from build123d import *

# Parameters (mm, degrees)
F0_W      = 50.8
F0_H      = 57.15
F1_DEPTH  = 3.175
F2_W      = 50.8
F2_H      = 3.175
F3_DEPTH  = 88.9
F4_W      = 50.8
F4_H      = 3.175
F5_DEPTH  = 88.9
F6_W      = 50.8
F6_H      = 88.9
F7_DEPTH  = 3.175
F8_W      = 57.15
F8_H      = 92.075
F9_DEPTH  = 3.175
F11_W     = 44.45
F11_H     = 3.175
F12_DEPTH = 88.9
F10_W     = 3.175
F10_H     = 50.8
F13_DEPTH = 88.9


with BuildPart() as f1:
    # F0 (on Top) → F1 (new body)
    with BuildSketch(Plane.XY):
        Rectangle(F0_W, F0_H)
    extrude(amount=F1_DEPTH)

    # F2 (on face) → F3 (join)
    with BuildSketch(Plane.XY.offset(3.175)):
        with Locations((0, 26.9875)):
            Rectangle(F2_W, F2_H)
    extrude(amount=F3_DEPTH)

    # F4 (on face) → F5 (join)
    with BuildSketch(Plane.XY.offset(3.175)):
        with Locations((0, -26.9875)):
            Rectangle(F4_W, F4_H)
    extrude(amount=F5_DEPTH)

    # F6 (on face) → F7 (join)
    with BuildSketch(Plane(origin=(-25.4, 0, 0), x_dir=(0, -1, 0), z_dir=(-1, 0, 0))):
        with Locations((0, 47.625)):
            Rectangle(F6_W, F6_H)
    extrude(amount=-F7_DEPTH)

    # F8 (on face) → F9 (join)
    with BuildSketch(Plane.YZ.offset(25.4)):
        with Locations((0, 46.0375)):
            Rectangle(F8_W, F8_H)
    extrude(amount=-F9_DEPTH)

    # F11 (on face) → F12 (join)
    with BuildSketch(Plane.XY.offset(3.175)):
        Rectangle(F11_W, F11_H)
    extrude(amount=F12_DEPTH)

    # F10 (on face) → F13 (join)
    with BuildSketch(Plane.XY.offset(3.175)):
        Rectangle(F10_W, F10_H)
    extrude(amount=F13_DEPTH)


solid = f1.part
Can you work these out from the model? Positions are in its coordinate system, mm. A direction names the side the tool comes from. Give positions to 0.01 mm unless a question says otherwise; leave off trailing zeros. Loops run counter-clockwise (first coordinate to the right, second up) from the corner with the lowest first, then second, coordinate; pieces in that order, holes last. Notation, with made-up numbers: (60.25, -9.75) -> (65.25, -9.75) arc R14 ccw to (65.25, 9.25) -> close; hole circle Ø5 at (46, -10). An arc over 180 degrees is marked (long way). Return JSON: item names as keys, results as strings.
Q1. On a 3-axis mill with a long thin cutter (end or side, diameter ignored), from which of +Z, -Z, +X, -X, +Y, -Y can I reach the whole of each face in a straight line? I mean faces 1 (the face through (-1.588, 13, 47)), 2 (the face through (0, -28.575, 45)). Say none if no direction works.
Checks:
{"face 1": "+Z", "face 2": "+Z, -Z, +X, -X, -Y"}
Q2. I want a section at A-A, the plane z = 83. List the corners of the cut face in (x, y) for me (1 decimal).
Checks:
{"outline": "(-25.4, -28.6) -> (25.4, -28.6) -> (25.4, 28.6) -> (-25.4, 28.6) -> close; hole (-22.2, -25.4) -> (-1.6, -25.4) -> (-1.6, -1.6) -> (-22.2, -1.6) -> close; hole (-22.2, 1.6) -> (-1.6, 1.6) -> (-1.6, 25.4) -> (-22.2, 25.4) -> close; hole (1.6, -25.4) -> (22.2, -25.4) -> (22.2, -1.6) -> (1.6, -1.6) -> close; hole (1.6, 1.6) -> (22.2, 1.6) -> (22.2, 25.4) -> (1.6, 25.4) -> close"}
Q3. I want a section at C-C, the plane x = -3. List the corners of the cut face in (y, z) for me (1 decimal), then the cut area to 3 significant figures.
Checks:
{"outline": "(-28.6, 0) -> (28.6, 0) -> (28.6, 92.1) -> (25.4, 92.1) -> (25.4, 3.2) -> (1.6, 3.2) -> (1.6, 92.1) -> (-1.6, 92.1) -> (-1.6, 3.2) -> (-25.4, 3.2) -> (-25.4, 92.1) -> (-28.6, 92.1) -> close", "area": "1,030 mm2"}
Q4. I need wall thicknesses on probe 1 along X at (y, z) = (-12.5, 65) (1 decimal); probe 2 along Y at (x, z) = (4.5, 7) (1 decimal); probe 3 along Z at (x, y) = (-4, -10) (3 decimals). Which ranges of each line are inside material? Lowest first, please.
Checks:
{"probe 1": "x = -25.4 to -22.2, -1.6 to 1.6, 22.2 to 25.4", "probe 2": "y = -28.6 to -25.4, -1.6 to 1.6, 25.4 to 28.6", "probe 3": "z = 0 to 3.175"}
Q5. For pin 1 Ø6 at (x, y) = (-9, 11.5) entering from +Z (3 decimals), with a flat end and sliding along its axis, tell me the tip position at first contact or that it passes through.
Checks:
{"pin 1": "stops at z = 3.175"}
Q6. We'd pull the mould along X, two halves only. Please class faces 3 (the face through (22.225, -14, 48)), 4 (the face through (0, 7, 92.075)), 5 (the face through (-25.4, 0, 47)): released by +X, released by -X, zero draft, split by the parting line, or undercut.
Checks:
{"face 3": "undercut", "face 4": "zero draft", "face 5": "released by -X"}
Q7. I want a section at B-B, the plane y = 14.5. List the corners of the cut face in (x, z) for me (1 decimal), then the cut area to 3 significant figures.
Checks:
{"outline": "(-25.4, 0) -> (25.4, 0) -> (25.4, 92.1) -> (22.2, 92.1) -> (22.2, 3.2) -> (1.6, 3.2) -> (1.6, 92.1) -> (-1.6, 92.1) -> (-1.6, 3.2) -> (-22.2, 3.2) -> (-22.2, 92.1) -> (-25.4, 92.1) -> close", "area": "1,010 mm2"}
